from build123d import *

# Parameters (mm, degrees)
SKETCH1_R           = 14
SKETCH1_R_2         = 3.125
BOSS_EXTRUDE1_DEPTH = 4
FILLET1_R           = 12
CUT_EXTRUDE2_DEPTH  = 10


with BuildPart() as part:
    # Sketch1 → Boss-Extrude1 (new body)
    with BuildSketch(Plane(origin=(0, 0, 0), x_dir=(1, 0, 0), z_dir=(0, 1, 0))):
        with BuildLine():
            Line((-49.477267507, 24), (0, 24))
            ThreePointArc((0, 24), (7.353702178, 22.845635563), (14, 19.49358869))
            Line((14, 19.49358869), (14, 49.477267507))
            ThreePointArc((14, 49.477267507), (19, 54.477267507), (24, 49.477267507))
            Line((24, 49.477267507), (24, 0))
            ThreePointArc((24, 0), (22.845635563, -7.353702178), (19.49358869, -14))
            Line((19.49358869, -14), (49.477267507, -14))
            ThreePointArc((49.477267507, -14), (54.477267507, -19), (49.477267507, -24))
            Line((49.477267507, -24), (0, -24))
            ThreePointArc((0, -24), (-7.353702178, -22.845635563), (-14, -19.49358869))
            Line((-14, -19.49358869), (-14, -49.477267507))
            ThreePointArc((-14, -49.477267507), (-19, -54.477267507), (-24, -49.477267507))
            Line((-24, -49.477267507), (-24, 0))
            ThreePointArc((-24, 0), (-22.845635563, 7.353702178), (-19.49358869, 14))
            Line((-19.49358869, 14), (-49.477267507, 14))
            ThreePointArc((-49.477267507, 14), (-54.477267507, 19), (-49.477267507, 24))
        make_face()
        with Locations(Location((0, 0, 0), (0, 0, 270))):
            Circle(SKETCH1_R, mode=Mode.SUBTRACT)
        with Locations(Location((-19, -49.477267507, 0), (0, 0, 270))):
            Circle(SKETCH1_R_2, mode=Mode.SUBTRACT)
        with Locations(Location((-49.477267507, 19, 0), (0, 0, 270))):
            Circle(SKETCH1_R_2, mode=Mode.SUBTRACT)
        with Locations(Location((19, 49.477267507, 0), (0, 0, 270))):
            Circle(SKETCH1_R_2, mode=Mode.SUBTRACT)
        with Locations(Location((49.477267507, -19, 0), (0, 0, 270))):
            Circle(SKETCH1_R_2, mode=Mode.SUBTRACT)
    extrude(amount=BOSS_EXTRUDE1_DEPTH)

    # Fillet1
    fillet1_edges = [part.edges().sort_by_distance(p)[0] for p in [
        (-19.49358869, 2, -14),
        (14, 2, -19.49358869),
        (19.49358869, 2, 14),
        (-14, 2, 19.49358869),
    ]]
    fillet(fillet1_edges, radius=FILLET1_R)

    # Sketch3 → Cut-Extrude2 (cut)
    with BuildSketch(Plane(origin=(0, 4, 0), x_dir=(1, 0, 0), z_dir=(0, 1, 0))):
        Polygon((9.585169941, 18.038972177), (8.882922363, 13.941796523), (12.080056774, 11.285044454), (15.979438763, 12.725468039), (16.681686341, 16.822643693), (13.48455193, 19.479395762), align=None)
        Polygon((-15.979438763, -12.725468039), (-16.681686341, -16.822643693), (-13.48455193, -19.479395762), (-9.585169941, -18.038972177), (-8.882922363, -13.941796523), (-12.080056774, -11.285044454), align=None)
    extrude(amount=-CUT_EXTRUDE2_DEPTH, mode=Mode.SUBTRACT)


solid = part.part
Work out the finished part from the listing and answer in its coordinate system (mm). A direction names the side the tool comes from. Round coordinates to 2 decimals unless told otherwise and drop trailing zeros. Loops run counter-clockwise (first coordinate to the right, second up) from the corner with the lowest first, then second, coordinate; pieces in that order, holes last. Notation, with made-up numbers: (43, 15) - (90, 15) arc R17 ccw to (90, 26) - close; hole circle Ø10 at (25.25, 85). An arc over 180 degrees is marked (long way). Use one line per item in the form item = value. Start each with the question number.
(1) Consider line 1 (Z direction, x = 5, y = 3.6); line 2 (Z direction, x = -3.5, y = 2.2); line 3 (Z direction, x = -44, y = 1.3). Determine where each line is inside the solid, lowest interval first.
(2) Find section B-B on z = 10. Determine the outline of the cut face in (x, y), and give its area (3 significant figures).
(3) Which of the six approach directions +Z, -Z, +X, -X, +Y, -Y give full straight-line access (tool end or side, diameter ignored) to faces 1 (the face through (-8, 4, 12)), 2 (the face through (14.002, 2.028, -11.995)), 3 (the face through (-8, 0, 12)), 4 (the face through (-43, 2, -14)), 5 (the face through (43, 2, 14))?
(4) Find section C-C on y = 1.4. Give the number of separate pieces and of enclosed holes in the cut face, and give its area (3 significant figures).
(5) Determine the mould class of faces 6 (the face through (-18.89, 1.972, 54.476)), 7 (the face through (-16.326, 2.028, 14.745)), 8 (the face through (18.89, 1.972, -54.476)), 9 (the face through (54.476, 1.972, 18.89)) for opening direction Z: +Z half, -Z half, draft (parallel to the pull), parting line (faces both ways), or undercut.
(6) Flat-ended cylindrical pins translate along their axes: P1, Ø1.2, axis at y = 1.5, z = -19, coming from the +X side; P2, Ø10, axis at x = -19, z = 49.48, coming from the +Y side; P3, Ø2, axis at x = -40.5, y = 2.5, coming from the +Z side; P4, Ø2, axis at y = 1.5, z = 7.5, coming from the +X side. Find the tip coordinate at first contact, or state that the pin passes through.
(7) Find section D-D on x = 43.5. Determine the outline of the cut face in (y, z), and give its area (3 significant figures).
(8) Find section A-A on x = 19. Determine the outline of the cut face in (y, z), and give its area (3 significant figures).
Answer list:
q1.line_1 = -24.33 to -13.08, 13.08 to 24
q1.line_2 = -24 to -13.56, 13.56 to 24.04
q1.line_3 = -24 to -14
q2.outline = (-24, 0) - (-9.8, 0) - (-9.8, 4) - (-24, 4) - close; (9.8, 0) - (27, 0) - (27, 4) - (9.8, 4) - close
q2.area = 126 mm^2
q3.face_1 = +Z, -Z, +X, -X, +Y
q3.face_2 = +Y, -Y
q3.face_3 = +Z, -Z, +X, -X, -Y
q3.face_4 = +Z, -X, +Y, -Y
q3.face_5 = -Z, +X, +Y, -Y
q4.separate_pieces = 1
q4.enclosed_holes = 7
q4.area = 2,770 mm^2
q5.face_6 = +Z half
q5.face_7 = undercut
q5.face_8 = -Z half
q5.face_9 = parting line
q6.P1 = 24
q6.P2 = 4
q6.P3 = -14
q6.P4 = 25.86
q7.outline = (0, 14) - (4, 14) - (4, 24) - (0, 24) - close
q7.area = 40.0 mm^2
q8.outline = (0, -54.48) - (4, -54.48) - (4, -52.6) - (0, -52.6) - close; (0, -46.35) - (4, -46.35) - (4, 24) - (0, 24) - close
q8.area = 289 mm^2
